```python
from build123d import *

# Parameters (mm, degrees)
EXTRUDE_L_DEPTH        = 15
EXTRUDE_951_DEPTH      = 15
FILLET_1044_R          = 5
SKETCH_1306_R          = 1.5
CUT_EXTRUDE_1314_DEPTH = 251.162599761


with BuildPart() as part:
    # Эскиз l → l (new body)
    with BuildSketch(Plane(origin=(0, 0, 0), x_dir=(1, 0, 0), z_dir=(0, 1, 0))):
        with BuildLine():
            Line((0, 163.701923077), (0, 200))
            Line((0, 200), (88.622884615, 200))
            Line((88.622884615, 200), (88.622884615, 51.682692308))
            add(Edge.make_bspline(
                [(88.622884615, 51.682692308), (88.584324136, 49.498745129), (89.03409536, 46.314042521), (90.756066544, 42.548836596), (92.543680506, 40.272944728), (94.800293255, 38.479885865), (98.492933692, 36.6691907), (101.687793554, 36.288646199), (103.84724359, 36.298076923)],
                knots=[0, 0, 0, 0, 0.266770811, 0.385688366, 0.501833832, 0.616701353, 0.734856032, 1, 1, 1, 1], degree=3))
            Line((103.84724359, 36.298076923), (149.520320513, 36.298076923))
            Line((149.520320513, 36.298076923), (149.520320513, 0))
            Line((149.520320513, 0), (99.680576923, 0))
            add(Edge.make_bspline(
                [(99.680576923, 0), (95.787985552, 0.056561193), (90.049186966, 0.354248464), (82.756449757, 1.913423248), (77.722410387, 3.420669789), (73.047421178, 5.435773635), (68.65960796, 7.842675126), (64.657079117, 10.74400138), (60.988860255, 14.046426407), (57.696300151, 17.73067833), (54.833554235, 21.805264076), (52.441129709, 26.224868693), (50.453789108, 30.958007277), (48.934002029, 36.035784324), (47.490582867, 43.441868234), (47.022391454, 49.220591435), (47.076410256, 53.165064103)],
                knots=[0, 0, 0, 0, 0.137920176, 0.202111555, 0.263363656, 0.323455843, 0.381806019, 0.440003085, 0.497856099, 0.556060831, 0.614368942, 0.673546606, 0.733454771, 0.79561061, 0.860632327, 1, 1, 1, 1], degree=3))
            Line((47.076410256, 53.165064103), (47.076410256, 153.701923077))
            ThreePointArc((47.076410256, 153.701923077), (44.147478068, 160.772990889), (37.076410256, 163.701923077))
            Line((37.076410256, 163.701923077), (0, 163.701923077))
        make_face()
    extrude(amount=EXTRUDE_L_DEPTH)

    # Sketch 848 → Extrude 951 (add)
    with BuildSketch(Plane(origin=(0, 0, 0), x_dir=(1, 0, 0), z_dir=(0, 1, 0))):
        with BuildLine():
            Line((10, 176.8490385), (52.853237, 176.8490385))
            ThreePointArc((52.853237, 176.8490385), (59.924304812, 173.920106312), (62.853237, 166.8490385))
            Line((62.853237, 166.8490385), (62.853237, 49.040393573))
            ThreePointArc((62.853237, 49.040393573), (73.181783835, 23.845809353), (98.223159353, 13.151162754))
            ThreePointArc((98.223159353, 13.151162754), (98.368899816, 13.149569571), (98.514648019, 13.1490385))
            Line((98.514648019, 13.1490385), (139.520321, 13.1490385))
            Line((139.520321, 13.1490385), (139.520321, 23.1490385))
            Line((139.520321, 23.1490385), (98.514648019, 23.1490385))
            ThreePointArc((98.514648019, 23.1490385), (98.441773917, 23.149304035), (98.368903686, 23.150100627))
            ThreePointArc((98.368903686, 23.150100627), (80.304193656, 30.865159632), (72.853237, 49.040393573))
            Line((72.853237, 49.040393573), (72.853237, 166.8490385))
            ThreePointArc((72.853237, 166.8490385), (66.995372624, 180.991174124), (52.853237, 186.8490385))
            Line((52.853237, 186.8490385), (10, 186.8490385))
            Line((10, 186.8490385), (10, 176.8490385))
        make_face()
    extrude(amount=-EXTRUDE_951_DEPTH)

    # Fillet 1044
    fillet_1044_edges = [part.edges().sort_by_distance(p)[0] for p in [
        (139.520321, -7.5, -13.1490385),
        (139.520321, -7.5, -23.1490385),
        (10, -7.5, -176.8490385),
        (10, -7.5, -186.8490385),
    ]]
    fillet(fillet_1044_edges, radius=FILLET_1044_R - 0.0001)  # a hair under: the kernel refuses the full size

    # Sketch 1306 → Cut-Extrude 1314 (cut, through all)
    with BuildSketch(Plane(origin=(0, 0, 0), x_dir=(1, 0, 0), z_dir=(0, 1, 0))):
        with Locations(Location((15, 181.849039, 0), (0, 0, 270))):
            Circle(SKETCH_1306_R)
        with Locations(Location((67.853237, 100, 0), (0, 0, 270))):
            Circle(SKETCH_1306_R)
        with Locations(Location((134.52, 18.149039, 0), (0, 0, 270))):
            Circle(SKETCH_1306_R)
    extrude(amount=-CUT_EXTRUDE_1314_DEPTH, mode=Mode.SUBTRACT)


solid = part.part
```
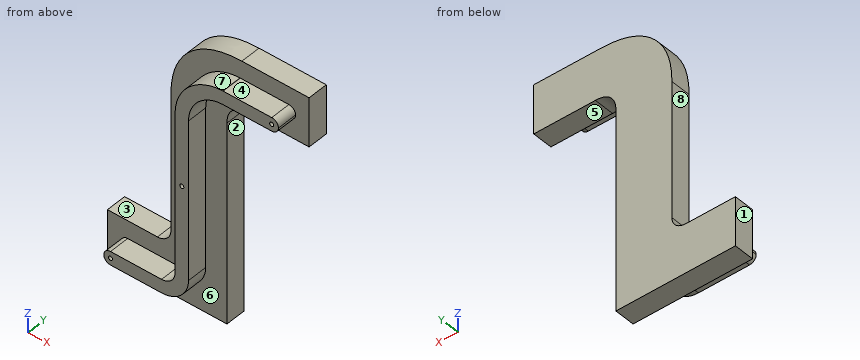
Check sheet for the modelled part. Datum: model origin and axes. Units: mm. Face numbers are marked on the shaded views. A direction names the side the tool comes from. Round coordinates to 2 decimals unless told otherwise and drop trailing zeros. Order: outer loops, then holes, each group sorted by start corner. A loop starts at its lowest first (then second) coordinate and runs counter-clockwise, first axis right, second up.
1) Scan lines: line 1 (X direction, y = -11.5, z = -100); line 2 (Z direction, x = 31, y = -10.5); line 3 (Y direction, x = 8.5, z = -186.5). Record each from-to range of solid material in increasing order.
2) Tool access check on the marked faces 4, 5, 6, 7 and 8. Record the directions out of +Z, -Z, +X, -X, +Y, -Y that give a thin tool (end or side, any length) a straight path to the whole face; none if there is none.
3) Section check A-A (z = -92.5). Record the boundary of the cut face in (x, y).
4) Go/stop test with flat-tipped pins: pin 1 Ø7.5 at (x, y) = (117, -7) entering from +Z; pin 2 Ø16.5 at (y, z) = (-8, -93.5) entering from +X; pin 3 Ø5 at (x, y) = (85, 2.5) entering from +Z. Record where each tip stops, or that it passes through.
5) Section check B-B (y = -4). Give the number of separate pieces and of enclosed holes in the cut face, and give its area (3 significant figures).
6) Mould release check, pull along X, two halves, no side actions. Record for the marked faces 1, 2 and 3: +X half, -X half, draft (parallel to the pull), parting line (faces both ways), or undercut.
Result:
1. line 1: x = 62.85 to 66.35, 69.35 to 72.85
1. line 2: z = -186.85 to -176.85
1. line 3: y = 0 to 15
2. face 4: +Z, +X, -X, -Y
2. face 5: -Z, +X, +Y, -Y
2. face 6: -Y
2. face 7: +Z, -X, -Y
2. face 8: +Z, -X, +Y, -Y
3. outline: (47.08, 0) - (62.85, 0) - (62.85, -15) - (72.85, -15) - (72.85, 0) - (88.62, 0) - (88.62, 15) - (47.08, 15) - close
4. pin 1: stops at z = -13.15
4. pin 2: stops at x = 88.62
4. pin 3: stops at z = -0.97
5. separate pieces: 1
5. enclosed holes: 3
5. area: 2,690 mm2
6. face 1: -X half
6. face 2: +X half
6. face 3: draft
